The listing builds one solid part. Answer for the finished solid, in the listing's coordinates (mm). A direction names the side the tool comes from. Coordinates: 2 decimals unless noted, no trailing zeros. Order: outer loops, then holes, each group sorted by start corner. A loop starts at its lowest first (then second) coordinate and runs counter-clockwise, first axis right, second up. Notation, with made-up numbers: (89, 0.25) -> (109, 0.25) arc R32 cw to (109, 36.25) -> close; hole circle Ø3 at (83, -33.5). An arc over 180 degrees is marked (long way). Write item = value, one per line.
from build123d import *

# Parameters (mm, degrees)
F0_W     = 55.000004
F0_H     = 70.000004
F0_W_2   = 45
F0_H_2   = 60
F1_DEPTH = 5
F2_W     = 55.000004
F2_H     = 70.000004
F3_DEPTH = 5
F4_R     = 5
F5_DEPTH = 0.5


with BuildPart() as f1:
    # F0 (on Top) → F1 (new body)
    with BuildSketch(Plane.XY):
        Rectangle(F0_W, F0_H)
        Rectangle(F0_W_2, F0_H_2, mode=Mode.SUBTRACT)
    extrude(amount=F1_DEPTH)

    # F2 (on face) → F3 (join)
    with BuildSketch(Plane(origin=(0, 0, 0), x_dir=(1, 0, 0), z_dir=(0, 0, -1))):
        Rectangle(F2_W, F2_H)
    extrude(amount=F3_DEPTH)

    # F4 (on face) → F5 (join)
    with BuildSketch(Plane(origin=(0, 0, -5), x_dir=(1, 0, 0), z_dir=(0, 0, -1))):
        with Locations((-27.500002, 35.000002)):
            Circle(F4_R)
        with Locations((27.500002, 35.000002)):
            Circle(F4_R)
        with Locations((27.500002, -35.000002)):
            Circle(F4_R)
        with Locations((-27.500002, -35.000002)):
            Circle(F4_R)
    extrude(amount=-F5_DEPTH)


solid = f1.part
Q1. Section A-A, the plane z = 2 is taken. Give the vertices of the cut face in (x, y).
The answers:
outline = (-27.5, -35) -> (27.5, -35) -> (27.5, 35) -> (-27.5, 35) -> close; hole (-22.5, -30) -> (22.5, -30) -> (22.5, 30) -> (-22.5, 30) -> close
Q2. Each of these flat-tipped pins is pushed along its axis until it touches: pin 1 Ø5.5 at (y, z) = (2, 2) entering from +X; pin 2 Ø11 at (x, y) = (30, -37.5) entering from +Z; pin 3 Ø5 at (x, z) = (13.5, 1) entering from -Y; pin 4 Ø4 at (x, z) = (5, 3.5) entering from +Y. Where does it stop, or does it pass through?
The answers:
pin_1 = 27.5
pin_2 = 5
pin_3 = -35
pin_4 = 35
Q3. A tool of negligible diameter and unlimited length cuts with its end or side. For faces 5 (the face through (30.92, 38.65, -4.75)), 6 (the face through (0, 0, 0)), from which of +Z, -Z, +X, -X, +Y, -Y can it reach the whole face along a straight path? Write none if from no direction.
The answers:
face_5 = +Z, -Z
face_6 = +Z
Q4. Find the intervals of material crossed by line 1 along Y through (x, z) = (-14.5, 3.75); line 2 along X through (y, z) = (-4, 0.25); line 3 along Y through (x, z) = (13, -1), in increasing order.
The answers:
line_1 = -35 to -30, 30 to 35
line_2 = -27.5 to -22.5, 22.5 to 27.5
line_3 = -35 to 35
Q5. Section C-C, the plane x = -3 is taken. Give the vertices of the cut face in (y, z), plus the area to 3 significant figures.
The answers:
outline = (-35, -5) -> (35, -5) -> (35, 5) -> (30, 5) -> (30, 0) -> (-30, 0) -> (-30, 5) -> (-35, 5) -> close
area = 400 mm2
Q6. The mould has two halves that part along Y. Classify faces 1 (the face through (22.5, 0, 2)), 2 (the face through (29, -36, -4.5)), 3 (the face through (0, -35, 0)), 4 (the face through (0, 30, 2)): released by +Y, released by -Y, zero draft, split by the parting line, or undercut.
The answers:
face_1 = undercut
face_2 = zero draft
face_3 = released by -Y
face_4 = undercut
Q7. Section B-B, the plane y = -5 is taken. Give the vertices of the cut face in (x, z), plus the area to 3 significant figures.
The answers:
outline = (-27.5, -5) -> (27.5, -5) -> (27.5, 5) -> (22.5, 5) -> (22.5, 0) -> (-22.5, 0) -> (-22.5, 5) -> (-27.5, 5) -> close
area = 325 mm2
Q8. Section D-D, the plane z = -3 is taken. Give the vertices of the cut face in (x, y), plus the area to 3 significant figures.
The answers:
outline = (-27.5, -35) -> (27.5, -35) -> (27.5, 35) -> (-27.5, 35) -> close
area = 3,850 mm2
